```python
from build123d import *

# Parameters (mm, degrees)
SKETCH1_R           = 7
SKETCH1_R_2         = 6
BOSS_EXTRUDE1_DEPTH = 400
CUT_EXTRUDE1_DEPTH  = 7


with BuildPart() as part:
    # Sketch1 → Boss-Extrude1 (new body)
    with BuildSketch(Plane(origin=(0, 0, 0), x_dir=(1, 0, 0), z_dir=(0, 1, 0))):
        with Locations(Location((0, 0, 0), (0, 0, 270))):
            Circle(SKETCH1_R)
        with Locations(Location((0, 0, 0), (0, 0, 270))):
            Circle(SKETCH1_R_2, mode=Mode.SUBTRACT)
    extrude(amount=BOSS_EXTRUDE1_DEPTH)

    # Sketch3 → Cut-Extrude1 (cut)
    with BuildSketch(Plane.XY.offset(-10)):
        Polygon((-6, 15), (-6, 1), (0, 1), (8, 1), (8, 15), align=None)
    extrude(amount=CUT_EXTRUDE1_DEPTH, mode=Mode.SUBTRACT)


solid = part.part
```
Work out the finished part from the listing and answer in its coordinate system (mm). Round coordinates to 2 decimals unless told otherwise and drop trailing zeros. Write each loop counter-clockwise with the first axis right and the second up, starting at its lowest first coordinate (ties: lowest second). Pieces come first, ordered by that corner, then holes.
1) A cutting plane is placed at C-C on y = 267. Determine the outline of the cut face in (x, z).
2) Flat-ended cylindrical pins translate along their axes: P1, Ø1, axis at x = -2.5, y = 308.5, coming from the +Z side; P2, Ø1.5, axis at y = 259, z = 5, coming from the +X side; P3, Ø6, axis at x = -2, y = 309, coming from the -Z side; P4, Ø4, axis at x = 2.5, y = 344.5, coming from the +Z side. Find the tip coordinate at first contact, or state that the pin passes through.
3) A cutting plane is placed at A-A on x = 0. Determine the outline of the cut face in (y, z).
4) A cutting plane is placed at B-B on z = 1.25. Determine the outline of the cut face in (x, y).
5) Determine the mould class of faces 1 (the face through (2, 400, 6)), 2 (the face through (1.802, 197.2, 5.723)), 3 (the face through (-6.834, 197.2, -1.517)) for opening direction Z: pulls with the +Z half, pulls with the -Z half, needs draft (parallel to the pull), parting line crosses it, or undercut.
6) Consider probe 1 along Z at (x, y) = (0, 240.5); probe 2 along Y at (x, z) = (-1.25, -6). Determine where each line is inside the solid, lowest interval first.
Entries:
1. outline: circle Ø14 at (0, 0); hole circle Ø12 at (0, 0)
2. P1: stops at z = 6.71
2. P2: stops at x = 5.56
2. P3: stops at z = -7
2. P4: stops at z = 6.98
3. outline: (0, -7) - (1, -7) - (1, -6) - (0, -6) - close; (0, 6) - (400, 6) - (400, 7) - (0, 7) - close; (15, -7) - (400, -7) - (400, -6) - (15, -6) - close
4. outline: (-6.89, 0) - (-5.87, 0) - (-5.87, 400) - (-6.89, 400) - close; (5.87, 0) - (6.89, 0) - (6.89, 400) - (5.87, 400) - close
5. face 1: needs draft
5. face 2: undercut
5. face 3: parting line crosses it
6. probe 1: z = -7 to -6, 6 to 7
6. probe 2: y = 0 to 1, 15 to 400
